Autodesk Inventor part; units mm, degrees
ref_plane "Start Plane" through (0, 0, 7.6064) normal (0, 0, 1) x (1, 0, 0)
ref_plane "End Plane" through (0, 0, 93.0129) normal (0, 0, 1) x (1, 0, 0)
ref_plane "Work Plane5" through (4.0763, -50, 11.5058) normal (0.267, 0, -0.9637) x (-0.9637, 0, -0.267)
ref_plane "Start Plane" through (0, 0, 7.6064) normal (0, 0, 1) x (1, 0, 0)
ref_plane "End Plane" through (0, 0, 93.0129) normal (0, 0, 1) x (1, 0, 0)
sketch "Sketch" plane through (0, 0, 0) normal (0, 0, 1) x (1, 0, 0)
  line L0 (-10, -7) -> (-10, 7)
  line L1 (-7, 10) -> (7, 10)
  line L2 (10, 7) -> (10, -7)
  line L3 (7, -10) -> (-7, -10)
  arc A0 (-10, -7) -> (-7, -10) centre (-7, -7) ccw
  arc A1 (-7, 10) -> (-10, 7) centre (-7, 7) ccw
  arc A2 (10, 7) -> (7, 10) centre (7, 7) ccw
  arc A3 (7, -10) -> (10, -7) centre (7, -7) ccw
  arc A4 (-7, 8) -> (-8, 7) centre (-7, 7) ccw
  line L4 (-7, 8) -> (7, 8)
  arc A5 (8, 7) -> (7, 8) centre (7, 7) ccw
  line L5 (8, 7) -> (8, -7)
  arc A6 (7, -8) -> (8, -7) centre (7, -7) ccw
  line L6 (7, -8) -> (-7, -8)
  arc A7 (-8, -7) -> (-7, -8) centre (-7, -7) ccw
  line L7 (-8, -7) -> (-8, 7)
  line L8 (0, 14.8698) -> (0, -14.8698) construction
  line L9 (-14.8698, 0) -> (14.8698, 0) construction
  dimension "d7" = 3
  dimension "d10" = 20
  dimension "d11" = 20
  dimension "d12" = 2
  dimension "d15" = 10
  dimension "d16" = 10
extrude "Body" add sketch "Sketch" along normal up to surface (85.4065 mm away) from surface at 7.6064
sketch "Sketch3" plane through (0, 0, 0) normal (0, 0, 1) x (1, 0, 0)
  line L0 (0, 0) -> (10, 0)
ref_plane "Work Plane3" through (0, 0, 0) normal (0, -1, 0) x (1, 0, 0)
sketch "Sketch4" plane through (0, 0, 0) normal (0, -1, 0) x (1, 0, 0)
  line L0 (-2, 7.6064) -> (12, 7.6064)
  line L1 (-2, 93.0129) -> (12, 93.0129)
  dimension "d18" = 85.4065
ref_plane "Work Plane5" through (4.0763, -50, 11.5058) normal (0.267, 0, -0.9637) x (-0.9637, 0, -0.267)
split "Split2" plane through (4.0763, -50, 11.5058) removes the side toward (0.267, 0, -0.9637)
ref_plane "Work Plane6" through (0, 0, 93.0129) normal (0, 0, 1) x (1, 0, 0)
split "Split3" plane through (0, 0, 93.0129) removes the side toward (0, 0, 1)
ref_plane "Work Plane7" through (0, 10, 93.0129) normal (0, -0.7071, 0.7071) x (1, 0, 0)
split "Split4" plane through (0, 10, 93.0129) removes the side toward (0, -0.7071, 0.7071)
sketch "Sketch7" plane through (8, -7, 12.5928) normal (-1, 0, 0) x (0, 0, 1)
  point P0 (11.4871, 7)
hole "Hole3" at (8, 0, 24.0799) direction (1, 0, 0) diameter 6.6 depth 2
sketch "Sketch8" plane through (8, -7, 12.5928) normal (-1, 0, 0) x (0, 0, 1)
  point P0 (66.4871, 7)
hole "Hole4" at (8, 0, 79.0799) direction (1, 0, 0) diameter 6.6 depth 2
sketch "Sketch9" plane through (-10, -7, 7.6064) normal (-1, 0, 0) x (0, 0, 1)
  point P0 (71.4735, 7)
hole "Hole5" at (-10, 0, 79.0799) direction (1, 0, 0) diameter 6.6 end through all
sketch "Sketch10" plane through (-10, -7, 7.6064) normal (-1, 0, 0) x (0, 0, 1)
  point P0 (16.4735, 7)
hole "Hole6" at (-10, 0, 24.0799) direction (1, 0, 0) diameter 6.6 end through all
equation "\"d7\" = G_IR"
equation "\"d10\" = G_H"
equation "\"d11\" = G_W"
equation "\"d12\" = G_T"
equation "\"d15\" = 0.5 * d10"
equation "\"d16\" = 0.5 * d11"
equation "\"d3\" = G_L"
equation "\"G_W\" = 20"
equation "\"G_H\" = 20"
equation "\"G_T\" = 2"
equation "\"G_IR\" = 3"
equation "\"G_L\" = d18"
equation "\"G_OFFSET_START\" = -7.60639"
equation "\"d13\" = -G_OFFSET_START"
equation "\"d14\" = G_OFFSET_END + B_L"
equation "\"B_L\" = 83.01292"
properties part number "ISO 12633-2 - 20x20x2 - 85,41" material "Steel, Mild"
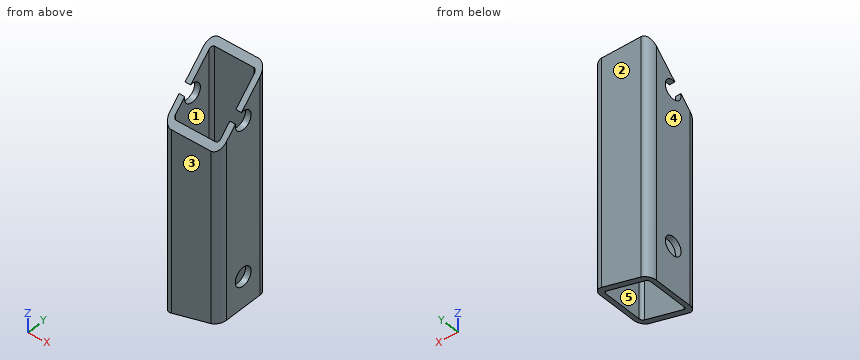
Geometry check sheet. Reference: the model listing, model coordinates, mm. Face numbers are marked on the shaded views. A direction names the side the tool comes from. Round coordinates to 2 decimals unless told otherwise and drop trailing zeros. Order: outer loops, then holes, each group sorted by start corner. A loop starts at its lowest first (then second) coordinate and runs counter-clockwise, first axis right, second up. Notation, with made-up numbers: M -30.5,69.5 L 9.5,69.5 A19 ccw 9.5,78.5 Z; hole C 73.5,87.25 d7. An arc over 180 degrees is marked long. Answer in a Markdown table with one row per item.
(1) Sectioned sample at D-D, the plane x = -5.5. Record the cut outline in (y, z), and give its area (3 significant figures).
Responses:
| item | result |
|---|---|
| outline | M -10,8.85 L -8,8.85 L -8,75.01 L -10,73.01 Z; M 8,8.85 L 10,8.85 L 10,93.01 L 8,91.01 Z |
| area | 297 mm² |
(2) Tool access check on the marked faces 1 and 2. Record the directions out of +Z, -Z, +X, -X, +Y, -Y that give a thin tool (end or side, any length) a straight path to the whole face; none if there is none.
Responses:
| item | result |
|---|---|
| face 1 | +Z, -Z |
| face 2 | +Z, -Z, +X, -X, +Y |
(3) Go/stop test with flat-tipped pins: P1, Ø6, axis at x = -7.5, y = -4.5, coming from the -Z side; P2, Ø5, axis at x = 8, y = -4.5, coming from the +Z side. Record where each tip stops, or that it passes through.
Responses:
| item | result |
|---|---|
| P1 | stops at z = 7.61 |
| P2 | stops at z = 79.79 |
(4) Scan lines: probe 1 along X at (y, z) = (-6, 61.5); probe 2 along Z at (x, y) = (8.8, 0). Record each from-to range of solid material in increasing order. Write a range as from..to.
Responses:
| item | result |
|---|---|
| probe 1 | x = -10..-8, 8..10 |
| probe 2 | z = 12.81..20.78, 27.38..75.78, 82.38..83.01 |
(5) Sectioned sample at A-A, the plane z = 57.5. Record the cut outline in (x, y).
Responses:
| item | result |
|---|---|
| outline | M -10,-7 A3 ccw -7,-10 L 7,-10 A3 ccw 10,-7 L 10,7 A3 ccw 7,10 L -7,10 A3 ccw -10,7 Z; hole M -8,-7 A1 ccw -7,-8 L 7,-8 A1 ccw 8,-7 L 8,7 A1 ccw 7,8 L -7,8 A1 ccw -8,7 Z |
(6) Sectioned sample at B-B, the plane x = 6. Record the cut outline in (y, z), and give its area (3 significant figures).
Responses:
| item | result |
|---|---|
| outline | M -10,12.04 L -8,12.04 L -8,75.01 L -10,73.01 Z; M 8,12.04 L 10,12.04 L 10,93.01 L 8,91.01 Z |
| area | 284 mm² |
(7) Draft check along Y on the marked faces 3, 4 and 5. Enter one of: released by +Y, released by -Y, zero draft, split by the parting line, or undercut.
Responses:
| item | result |
|---|---|
| face 3 | released by -Y |
| face 4 | zero draft |
| face 5 | undercut |
